CAD build for the part. Positions are in the model's coordinates, mm. Face numbers are marked on the shaded views. Coordinates: 2 decimals unless noted, no trailing zeros. Order: outer loops, then holes, each group sorted by start corner. A loop starts at its lowest first (then second) coordinate and runs counter-clockwise, first axis right, second up. Notation, with made-up numbers: M 34,-7 L 60,-7 A23 cw 60,25 Z; hole C 17.5,58.5 d2. An arc over 180 degrees is marked long. One line per item, written item: value.
from build123d import *

# Parameters (mm, degrees)
BOSS_EXTRUDE1_DEPTH = 210
FILLET2_R           = 15


with BuildPart() as part:
    # Sketch1 → Boss-Extrude1 (new body)
    with BuildSketch(Plane.XY):
        with BuildLine():
            Line((-60, 259.511669092), (-60, 246.811669092))
            ThreePointArc((-60, 246.811669092), (0, 254), (60, 246.811669092))
            Line((60, 246.811669092), (60, 259.511669092))
            ThreePointArc((60, 259.511669092), (0, 266.7), (-60, 259.511669092))
        make_face()
    extrude(amount=BOSS_EXTRUDE1_DEPTH)

    # Fillet2
    fillet2_edges = [part.edges().sort_by_distance(p)[0] for p in [
        (60, 253.161669092, 210),
        (60, 253.161669092, 0),
        (-60, 253.161669092, 0),
        (-60, 253.161669092, 210),
    ]]
    fillet(fillet2_edges, radius=FILLET2_R)


solid = part.part
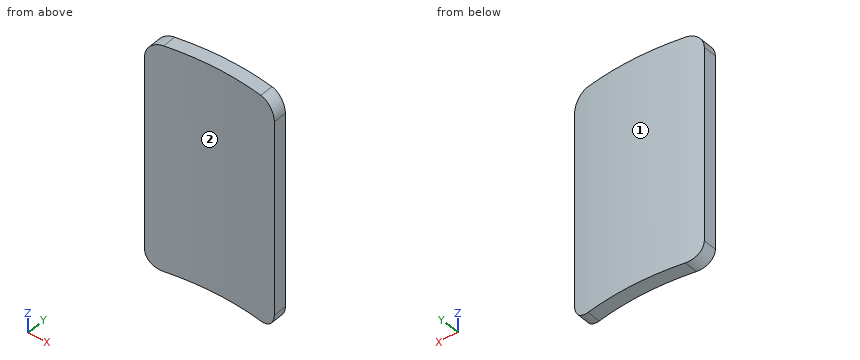
Q1. Pin check, flat tips, straight feed: pin 1 Ø6 at (x, z) = (-36.5, 115.5) entering from -Y; pin 2 Ø12 at (x, z) = (38, 154) entering from +Y. Stop position of each tip, or through.
Recorded:
pin 1: stops at y = 250.91
pin 2: stops at y = 264.68
Q2. Slice it at B-B (x = -48). List the corners of the cut face in (y, z), plus the area to 3 significant figures.
Recorded:
outline: M 249.42,0.3 L 262.12,0.3 L 262.12,209.7 L 249.42,209.7 Z
area: 2,660 mm^2
Q3. Mould opens along X. For the marked faces 1 and 2 say: released by +X, released by -X, zero draft, split by the parting line, or undercut.
Recorded:
face 1: split by the parting line
face 2: undercut
Q4. Slice it at A-A (z = 99.5). List the corners of the cut face in (x, y), plus the area to 3 significant figures.
Recorded:
outline: M -60,246.81 A254 cw 60,246.81 L 60,259.51 A254 ccw -60,259.51 Z
area: 1,520 mm^2
Q5. Drill centre lines: line 1 along Y through (x, z) = (-2.5, 80); line 2 along Y through (x, z) = (45, 133); line 3 along Z through (x, y) = (50.5, 249.75). Where is each one in solid material? Low to high.
Recorded:
line 1: y = 253.99 to 266.69
line 2: y = 249.98 to 262.68
line 3: z = 1.04 to 208.96
